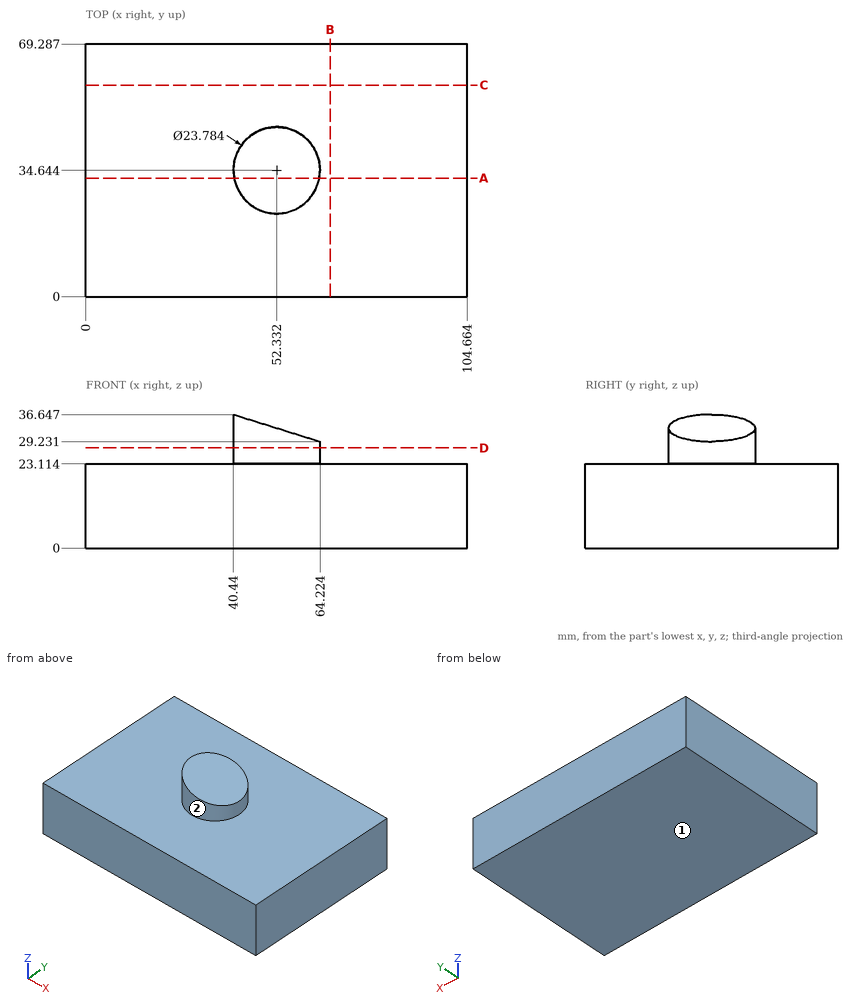
Geometry check sheet. Reference: drawing and pictorial views, mm from the part's lowest x, y, z. A direction names the side the tool comes from. Give positions to 0.01 mm unless a question says otherwise; leave off trailing zeros. Loops run counter-clockwise (first coordinate to the right, second up) from the corner with the lowest first, then second, coordinate; pieces in that order, holes last. Notation, with made-up numbers: (83, 3) -> (127, 3) arc R13 cw to (127, 20) -> close; hole circle Ø6 at (-37, 40). An arc over 180 degrees is marked (long way). Answer in a Markdown table with one row per item. Add a question column.
1) Set-up check for the marked faces 1 and 2: record each of +Z, -Z, +X, -X, +Y, -Y from which the full face is reachable in a straight line by a thin tool's end or side.
2) Cross-section at B-B on x = 67. Record the boundary of the cut face in (y, z) (1 decimal), and give its area (3 significant figures).
3) Cross-section at A-A on y = 32.5. Record the boundary of the cut face in (x, z) (1 decimal).
4) Gauge pin test, flat ends, axial feed: P1, Ø1, axis at y = 21, z = 25, coming from the +X side; P2, Ø2, axis at x = 19, y = 52, coming from the +Z side. Record the tip position at first contact, or that the pin passes through.
5) Material ranges on probe 1 along Z at (x, y) = (96, 20.5) (1 decimal); probe 2 along Z at (x, y) = (45, 30.5) (1 decimal); probe 3 along Y at (x, z) = (50.5, 25) (1 decimal), recorded low to high. Write a range as from..to.
6) Cross-section at C-C on y = 58. Record the boundary of the cut face in (x, z) (1 decimal).
7) Cross-section at D-D on z = 27.5. Record the boundary of the cut face in (x, y) (1 decimal), and give its area (3 significant figures).
Outcome:
| question | item | result |
|---|---|---|
| 1 | face 1 | -Z, +X, -X, +Y, -Y |
| 1 | face 2 | +Z |
| 2 | outline | (0, 0) -> (69.3, 0) -> (69.3, 23.1) -> (0, 23.1) -> close |
| 2 | area | 1,600 mm^2 |
| 3 | outline | (0, 0) -> (104.7, 0) -> (104.7, 23.1) -> (64, 23.1) -> (64, 29.3) -> (40.6, 36.6) -> (40.6, 23.1) -> (0, 23.1) -> close |
| 4 | P1 | passes through |
| 4 | P2 | stops at z = 23.11 |
| 5 | probe 1 | z = 0..23.1 |
| 5 | probe 2 | z = 0..35.2 |
| 5 | probe 3 | y = 22.9..46.4 |
| 6 | outline | (0, 0) -> (104.7, 0) -> (104.7, 23.1) -> (0, 23.1) -> close |
| 7 | outline | circle Ø23.8 at (52.3, 34.6) |
| 7 | area | 444 mm^2 |
